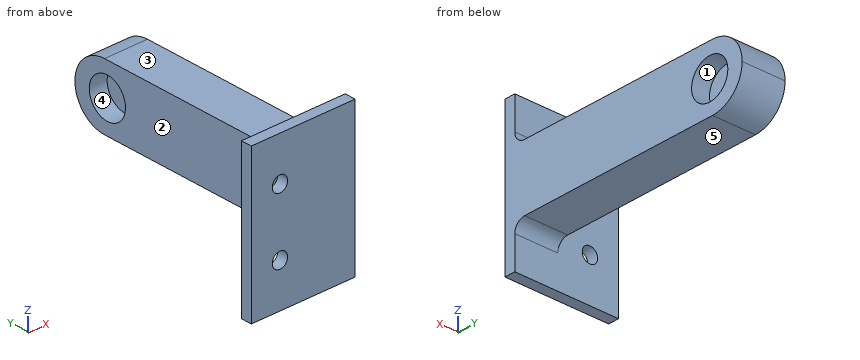
from build123d import *

# Parameters (mm, degrees)
SKETCH1_W            = 94
SKETCH1_H            = 42
BOSS_EXTRUDE1_DEPTH  = 3
SKETCH2_W            = 4
SKETCH2_H            = 42
BOSS_EXTRUDE2_DEPTH  = 47
SKETCH3_R            = 12.5
SKETCH3_R_2          = 1.6
CUT_EXTRUDE1_DEPTH   = 114.176852757
SKETCH4_W            = 42
SKETCH4_H            = 5
BOSS_EXTRUDE3_DEPTH  = 40
SKETCH5_W            = 42
SKETCH5_H            = 5
BOSS_EXTRUDE4_DEPTH  = 38
SKETCH7_W            = 42
SKETCH7_H            = 42
SKETCH7_W_2          = 44
BOSS_EXTRUDE6_DEPTH  = 5
SKETCH9_R            = 2.15
CUT_EXTRUDE2_DEPTH   = 149.731301346
SKETCH11_W           = 10
SKETCH11_H           = 18
BOSS_EXTRUDE7_DEPTH  = 20
SKETCH13_R           = 5.5
CUT_EXTRUDE3_DEPTH   = 169.988165266
BOSS_EXTRUDE11_DEPTH = 5
SKETCH23_W           = 10
SKETCH23_H           = 26
BOSS_EXTRUDE12_DEPTH = 50
CUT_EXTRUDE7_DEPTH   = 193.595430891
SKETCH25_W           = 10
SKETCH25_H           = 18
BOSS_EXTRUDE13_DEPTH = 20
SKETCH26_R           = 5.5
CUT_EXTRUDE8_DEPTH   = 193.595430891
SKETCH27_W           = 12
SKETCH27_H           = 18
BOSS_EXTRUDE14_DEPTH = 69
CUT_EXTRUDE10_START  = -5
SKETCH28_R           = 5.5
CUT_EXTRUDE10_DEPTH  = 5
SKETCH29_R           = 5.5
CUT_EXTRUDE11_DEPTH  = 5
FILLET4_R            = 9
FILLET3_R            = 3
SKETCH30_W           = 60
SKETCH30_H           = 42
SKETCH30_W_2         = 81
SKETCH30_H_2         = 100
CUT_EXTRUDE12_DEPTH  = 181.413414135
SKETCH31_W           = 2
SKETCH31_H           = 42
CUT_EXTRUDE13_DEPTH  = 10


# Some blends are built 0.0001 mm under size
with BuildPart() as part:
    # Sketch1 → Boss-Extrude1 (new body)
    with BuildSketch(Plane(origin=(0, 0, 0), x_dir=(1, 0, 0), z_dir=(0, 1, 0))):
        with Locations((47, -21)):
            Rectangle(SKETCH1_W, SKETCH1_H)
    extrude(amount=BOSS_EXTRUDE1_DEPTH)

    # Sketch2 → Boss-Extrude2 (add)
    with BuildSketch(Plane.XZ):
        with Locations((2, 21)):
            Rectangle(SKETCH2_W, SKETCH2_H)
        with Locations((92, 21)):
            Rectangle(SKETCH2_W, SKETCH2_H)
    extrude(amount=-BOSS_EXTRUDE2_DEPTH)

    # Sketch3 → Cut-Extrude1 (cut, through all)
    with BuildSketch(Plane(origin=(94, 0, 0), x_dir=(0, 0, -1), z_dir=(1, 0, 0))):
        with Locations((-21, 26)):
            Circle(SKETCH3_R)
        with Locations((-36.5, 41.5)):
            Circle(SKETCH3_R_2)
        with Locations((-5.5, 41.5)):
            Circle(SKETCH3_R_2)
        with Locations((-36.5, 10.5)):
            Circle(SKETCH3_R_2)
        with Locations((-5.5, 10.5)):
            Circle(SKETCH3_R_2)
    extrude(amount=-CUT_EXTRUDE1_DEPTH, mode=Mode.SUBTRACT)

    # Sketch4 → Boss-Extrude3 (add)
    with BuildSketch(Plane(origin=(94, 0, 0), x_dir=(0, 0, -1), z_dir=(1, 0, 0))):
        with Locations((-21, 2.5)):
            Rectangle(SKETCH4_W, SKETCH4_H)
    extrude(amount=BOSS_EXTRUDE3_DEPTH)

    # Sketch5 → Boss-Extrude4 (add)
    with BuildSketch(Plane.ZY):
        with Locations((21, 2.5)):
            Rectangle(SKETCH5_W, SKETCH5_H)
    extrude(amount=BOSS_EXTRUDE4_DEPTH)

    # Sketch7 → Boss-Extrude6 (add)
    with BuildSketch(Plane(origin=(0, 47, 0), x_dir=(1, 0, 0), z_dir=(0, 1, 0))):
        with Locations((-17, -21)):
            Rectangle(SKETCH7_W, SKETCH7_H)
        with Locations((112, -21)):
            Rectangle(SKETCH7_W_2, SKETCH7_H)
    extrude(amount=BOSS_EXTRUDE6_DEPTH)

    # Sketch9 → Cut-Extrude2 (cut, through all)
    with BuildSketch(Plane(origin=(0, 3, 0), x_dir=(1, 0, 0), z_dir=(0, 1, 0))):
        with Locations(Location((83, -20, 0), (0, 0, 270))):
            Circle(SKETCH9_R)
        with Locations(Location((65, -20, 0), (0, 0, 270))):
            Circle(SKETCH9_R)
        with Locations(Location((74, -11, 0), (0, 0, 270))):
            Circle(SKETCH9_R)
        with Locations(Location((74, -29, 0), (0, 0, 270))):
            Circle(SKETCH9_R)
        with Locations(Location((16, -12, 0), (0, 0, 270))):
            Circle(SKETCH9_R)
        with Locations(Location((16, -30, 0), (0, 0, 270))):
            Circle(SKETCH9_R)
        with Locations(Location((32, -12, 0), (0, 0, 270))):
            Circle(SKETCH9_R)
        with Locations(Location((32, -30, 0), (0, 0, 270))):
            Circle(SKETCH9_R)
    extrude(amount=-CUT_EXTRUDE2_DEPTH, mode=Mode.SUBTRACT)

    # Sketch11 → Boss-Extrude7 (add)
    with BuildSketch(Plane(origin=(0, 52, 0), x_dir=(1, 0, 0), z_dir=(0, 1, 0))):
        with Locations((-8, -21)):
            Rectangle(SKETCH11_W, SKETCH11_H)
        with Locations((107, -21)):
            Rectangle(SKETCH11_W, SKETCH11_H)
    extrude(amount=BOSS_EXTRUDE7_DEPTH)

    # Sketch13 → Cut-Extrude3 (cut, through all)
    with BuildSketch(Plane.ZY.offset(13)):
        with Locations((21, 62.15)):
            Circle(SKETCH13_R)
    extrude(amount=-CUT_EXTRUDE3_DEPTH, mode=Mode.SUBTRACT)

    # Sketch20 → Boss-Extrude11 (add)
    with BuildSketch(Plane.XY.offset(42)):
        Polygon((134, 0), (134, 52), (90, 52), (90, 0), (95, 0), (95, 20), (102, 26), (112, 26), (129, 20), (129, 0), align=None)
    extrude(amount=BOSS_EXTRUDE11_DEPTH)

    # Sketch23 → Boss-Extrude12 (add)
    with BuildSketch(Plane.XY.offset(47)):
        with Locations((107, 39)):
            Rectangle(SKETCH23_W, SKETCH23_H)
    extrude(amount=BOSS_EXTRUDE12_DEPTH)

    # Sketch24 → Cut-Extrude7 (cut, through all)
    with BuildSketch(Plane(origin=(112, 0, 0), x_dir=(0, 0, -1), z_dir=(1, 0, 0))):
        Polygon((-47, 26), (-97, 39), (-97, 26), align=None)
    extrude(amount=-CUT_EXTRUDE7_DEPTH, mode=Mode.SUBTRACT)

    # Sketch25 → Boss-Extrude13 (add)
    with BuildSketch(Plane(origin=(0, 52, 0), x_dir=(1, 0, 0), z_dir=(0, 1, 0))):
        with Locations((107, -71)):
            Rectangle(SKETCH25_W, SKETCH25_H)
    extrude(amount=BOSS_EXTRUDE13_DEPTH)

    # Sketch26 → Cut-Extrude8 (cut, through all)
    with BuildSketch(Plane(origin=(112, 0, 0), x_dir=(0, 0, -1), z_dir=(1, 0, 0))):
        with Locations((-71, 62.15)):
            Circle(SKETCH26_R)
    extrude(amount=-CUT_EXTRUDE8_DEPTH, mode=Mode.SUBTRACT)

    # Sketch27 → Boss-Extrude14 (add)
    with BuildSketch(Plane(origin=(0, 3, 0), x_dir=(1, 0, 0), z_dir=(0, 1, 0))):
        with Locations((47, -21)):
            Rectangle(SKETCH27_W, SKETCH27_H)
    extrude(amount=BOSS_EXTRUDE14_DEPTH)

    # Sketch28 → Cut-Extrude10 (cut)
    with BuildSketch(Plane(origin=(53, 0, 0), x_dir=(0, 0, -1), z_dir=(1, 0, 0)).offset(CUT_EXTRUDE10_START)):
        with Locations(Location((-21, 62.15, 0), (0, 0, 180))):
            Circle(SKETCH28_R)
    extrude(amount=CUT_EXTRUDE10_DEPTH, mode=Mode.SUBTRACT)

    # Sketch29 → Cut-Extrude11 (cut)
    with BuildSketch(Plane.ZY.offset(-41)):
        with Locations((21, 62.15)):
            Circle(SKETCH29_R)
    extrude(amount=-CUT_EXTRUDE11_DEPTH, mode=Mode.SUBTRACT)

    # Fillet4
    fillet4_edges = [part.edges().sort_by_distance(p)[0] for p in [
        (-8, 72, 12),
        (-8, 72, 30),
        (107, 72, 12),
        (107, 72, 30),
        (107, 72, 62),
        (107, 72, 80),
        (47, 72, 12),
        (47, 72, 30),
    ]]
    fillet(fillet4_edges, radius=FILLET4_R - 0.0001)  # a hair under: the kernel refuses the full size

    # Fillet3
    # the kernel refuses this fillet: 3 mm, written as the material it adds along each edge
    with BuildSketch(Plane(origin=(-3, 52, 30), x_dir=(0, 1, 0), z_dir=(-1, 0, 0)), Plane(origin=(112, 52, 80), x_dir=(0, 1, 0), z_dir=(-1, 0, 0))) as fillet3_piece_1:
        with BuildLine():
            CenterArc((FILLET3_R, -FILLET3_R), FILLET3_R, 90, 90)
            Line((0, -FILLET3_R), (0, 0))
            Line((0, 0), (FILLET3_R, 0))
        make_face()
    extrude(amount=10)
    with BuildSketch(Plane(origin=(-13, 52, 12), x_dir=(0, 0, -1), z_dir=(1, 0, 0)), Plane(origin=(112, 52, 30), x_dir=(0, 0, 1), z_dir=(-1, 0, 0)), Plane(origin=(102, 52, 12), x_dir=(0, 0, -1), z_dir=(1, 0, 0)), Plane(origin=(102, 52, 62), x_dir=(0, 0, -1), z_dir=(1, 0, 0))) as fillet3_piece_2:
        with BuildLine():
            CenterArc((FILLET3_R, FILLET3_R), FILLET3_R, 180, 90)
            Line((0, FILLET3_R), (0, 0))
            Line((0, 0), (FILLET3_R, 0))
        make_face()
    extrude(amount=10)
    with BuildSketch(Plane(origin=(95, 20, 42), x_dir=(0, -1, 0), z_dir=(0, 0, 1))) as fillet3_piece_3:
        with BuildLine():
            CenterArc((FILLET3_R * 0.45993492247, FILLET3_R), FILLET3_R, 220.601294645, 49.398705355)
            Line((-FILLET3_R * 0.299321679895, FILLET3_R * 0.349208626544), (0, 0))
            Line((0, 0), (FILLET3_R * 0.45993492247, 0))
        make_face()
    extrude(amount=5)
    with BuildSketch(Plane(origin=(102, 26, 42), x_dir=(-0.7592566023652966, -0.6507913734559685, 0), z_dir=(0, 0, 1))) as fillet3_piece_4:
        with BuildLine():
            CenterArc((FILLET3_R * 0.369924076215, FILLET3_R), FILLET3_R, 229.398705355, 40.601294645)
            Line((-FILLET3_R * 0.28086729724, FILLET3_R * 0.240743397635), (0, 0))
            Line((0, 0), (FILLET3_R * 0.369924076215, 0))
        make_face()
    extrude(amount=5)
    with BuildSketch(Plane(origin=(112, 26, 42), x_dir=(0.942990333582889, -0.3328201177351389, 0), z_dir=(0, 0, 1))) as fillet3_piece_5:
        with BuildLine():
            CenterArc((FILLET3_R * 0.171292729553, -FILLET3_R), FILLET3_R, 90, 19.440034828)
            Line((-FILLET3_R * 0.161527388182, -FILLET3_R * 0.0570096664171), (0, 0))
            Line((0, 0), (FILLET3_R * 0.171292729553, 0))
        make_face()
    extrude(amount=5)
    with BuildSketch(Plane(origin=(129, 20, 42), x_dir=(0, -1, 0), z_dir=(0, 0, 1))) as fillet3_piece_6:
        with BuildLine():
            CenterArc((FILLET3_R * 0.707515081019, -FILLET3_R), FILLET3_R, 90, 70.559965172)
            Line((-FILLET3_R * 0.235475252564, -FILLET3_R * 0.667179882265), (0, 0))
            Line((0, 0), (FILLET3_R * 0.707515081019, 0))
        make_face()
    extrude(amount=5)
    with BuildSketch(Plane(origin=(53, 3, 30), x_dir=(0, 0, 1), z_dir=(-1, 0, 0)), Plane(origin=(41, 3, 12), x_dir=(0, 0, -1), z_dir=(1, 0, 0))) as fillet3_piece_7:
        with BuildLine():
            CenterArc((FILLET3_R, FILLET3_R), FILLET3_R, 180, 90)
            Line((0, FILLET3_R), (0, 0))
            Line((0, 0), (FILLET3_R, 0))
        make_face()
    extrude(amount=12)
    # the kernel refuses this fillet: 3 mm, written as the material it takes off along each edge
    with BuildSketch(Plane(origin=(94.5, 52, 97), x_dir=(0, 0, -1), z_dir=(1, 0, 0))) as fillet3_2_piece_1:
        with BuildLine():
            CenterArc((FILLET3_R, -FILLET3_R), FILLET3_R, 90, 90)
            Line((0, -FILLET3_R), (0, 0))
            Line((0, 0), (FILLET3_R, 0))
        make_face()
    extrude(amount=25, mode=Mode.SUBTRACT)
    with BuildSketch(Plane(origin=(117.799354812, 39, 97), x_dir=(0, -0.25163385176495195, -0.9678225067882716), z_dir=(-1, 0, 0))) as fillet3_2_piece_2:
        with BuildLine():
            CenterArc((FILLET3_R * 0.773247308247, -FILLET3_R), FILLET3_R, 90, 75.425783802)
            Line((-FILLET3_R * 0.194575198541, -FILLET3_R * 0.748366148235), (0, 0))
            Line((0, 0), (FILLET3_R * 0.773247308247, 0))
        make_face()
    extrude(amount=21.598709624, mode=Mode.SUBTRACT)

    # Sketch30 → Cut-Extrude12 (cut, through all)
    with BuildSketch(Plane.XZ):
        with Locations((-8, 21)):
            Rectangle(SKETCH30_W, SKETCH30_H)
        with Locations((93.5, 50)):
            Rectangle(SKETCH30_W_2, SKETCH30_H_2)
    extrude(amount=-CUT_EXTRUDE12_DEPTH, mode=Mode.SUBTRACT)

    # Sketch31 → Cut-Extrude13 (cut)
    with BuildSketch(Plane(origin=(0, 3, 0), x_dir=(1, 0, 0), z_dir=(0, 1, 0))):
        with Locations((23, -21)):
            Rectangle(SKETCH31_W, SKETCH31_H)
    extrude(amount=-CUT_EXTRUDE13_DEPTH, mode=Mode.SUBTRACT)


solid = part.part
Build history of the part. All positions in model axes, mm. Face numbers are marked on the shaded views. A direction names the side the tool comes from. Round coordinates to 2 decimals unless told otherwise and drop trailing zeros. Write each loop counter-clockwise with the first axis right and the second up, starting at its lowest first coordinate (ties: lowest second). Pieces come first, ordered by that corner, then holes. Notation, with made-up numbers: (-14.75, -16) -> (40.25, -16) arc R5 ccw to (40.25, -8) -> close; hole circle Ø3 at (47.25, 0.25). An arc over 180 degrees is marked (long way). Write item = value, one per line.
(1) Flat gauge pins, fed straight in: pin 1 (4 mm diameter, centred on x = 37.5, z = 14.5, fed in from +Y); pin 2 (9 mm diameter, centred on y = 62.15, z = 21, fed in from +X); pin 3 (10 mm diameter, centred on y = 62.15, z = 21, fed in from -X). Where does each tip first touch, or does it go through?
Answer:
pin_1 = 3
pin_2 = 48
pin_3 = 46
(2) Band-saw the part on B-B (z = 11). Give the cut face in (x, y).
Answer:
outline = (24, 0) -> (30.1, 0) -> (30.1, 3) -> (24, 3) -> close; (33.9, 0) -> (53, 0) -> (53, 3.76) -> (41, 3.76) -> (41, 3) -> (33.9, 3) -> close
(3) Band-saw the part on C-C (x = 32). Give the cut face in (y, z).
Answer:
outline = (0, 0) -> (3, 0) -> (3, 9.85) -> (0, 9.85) -> close; (0, 14.15) -> (3, 14.15) -> (3, 27.85) -> (0, 27.85) -> close; (0, 32.15) -> (3, 32.15) -> (3, 42) -> (0, 42) -> close
(4) Probe L1, parallel to Z at x = 51.25, y = 62.15; L2, parallel to Y at x = 50.6, z = 21; L3, parallel to X at y = 1.8, z = 12. List the from-to ranges inside material, lowest first.
Answer:
L1 = 12 to 15.5, 26.5 to 30
L2 = 0 to 56.65, 67.65 to 72
L3 = 24 to 29.85, 34.15 to 53
(5) Tool access for the marked faces 1, 2, 3, 4 and 5: list every direction of +Z, -Z, +X, -X, +Y, -Y with a clear straight run to the whole face (end or side of a thin tool).
Answer:
face_1 = +X
face_2 = +Z, -Z, -X, +Y
face_3 = +Z, +X, -X, +Y
face_4 = -X
face_5 = -Z, +X, -X, +Y
(6) Band-saw the part on D-D (y = 62.15). Give the cut face in (x, z).
Answer:
outline = (41, 12) -> (53, 12) -> (53, 15.5) -> (48, 15.5) -> (48, 26.5) -> (53, 26.5) -> (53, 30) -> (41, 30) -> (41, 26.5) -> (46, 26.5) -> (46, 15.5) -> (41, 15.5) -> close
